Here's how the part is built. I have some questions about the finished solid (model axes, mm). Round coordinates to 2 decimals unless told otherwise and drop trailing zeros. Write each loop counter-clockwise with the first axis right and the second up, starting at its lowest first coordinate (ties: lowest second). Pieces come first, ordered by that corner, then holes. Notation, with made-up numbers: M 58,50.25 L 91,50.25 A18 ccw 91,74.25 Z; hole C 78.25,3 d7. An arc over 180 degrees is marked long. Write item = value, one per line. Start each with the question number.
(1) I need wall thicknesses on line 1 along Z through (x, y) = (0.75, 1237.5). Which ranges of the line are inside material? Lowest first, please.
(2) I want a section at B-B (z = 14.5). List the corners of the cut face in (x, y) for me, and give its area (3 significant figures).
(3) I want a section at A-A (x = -3.5). List the corners of the cut face in (y, z) for me, and give its area (3 significant figures).
```python
from build123d import *

# Parameters (mm, degrees)
SKETCH_1_W          = 25
SKETCH_1_H          = 50
EXTRUDE_1_DEPTH     = 1600
SKETCH_4_R          = 4
CUT_EXTRUDE_4_DEPTH = 550
CUT_EXTRUDE_5_DEPTH = 60


with BuildPart() as part:
    # Эскиз1 → Бобышка-Вытянуть1 (new body)
    with BuildSketch(Plane(origin=(0, 0, 0), x_dir=(1, 0, 0), z_dir=(0, 1, 0))):
        Rectangle(SKETCH_1_W, SKETCH_1_H)
    extrude(amount=EXTRUDE_1_DEPTH)

    # Эскиз4 → Вырез-Вытянуть4 (cut)
    with BuildSketch(Plane(origin=(12.5, 0, 0), x_dir=(0, 0, -1), z_dir=(1, 0, 0))):
        with Locations((0, 237.5)):
            Circle(SKETCH_4_R)
        with Locations((0, 762.5)):
            Circle(SKETCH_4_R)
        with Locations((0, 1237.5)):
            Circle(SKETCH_4_R)
        with Locations((0, 1525)):
            Circle(SKETCH_4_R)
    extrude(amount=-CUT_EXTRUDE_4_DEPTH, mode=Mode.SUBTRACT)

    # Эскиз5 → Вырез-Вытянуть5 (cut)
    with BuildSketch(Plane.XY.offset(25)):
        Polygon((-12.5, 1600), (-12.5, 1517.37698565), (12.5, 1596.12698565), (12.5, 1600), align=None)
    extrude(amount=-CUT_EXTRUDE_5_DEPTH, mode=Mode.SUBTRACT)


solid = part.part
```
Returned:
q1.line_1 = -25 to -4, 4 to 25
q2.outline = M -12.5,0 L 12.5,0 L 12.5,1596.13 L -12.5,1517.38 Z
q2.area = 38,900 mm²
q3.outline = M 0,-25 L 1545.73,-25 L 1545.73,25 L 0,25 Z; hole C 237.5,0 d8; hole C 762.5,0 d8; hole C 1237.5,0 d8; hole C 1525,0 d8
q3.area = 77,100 mm²
